Geometry check sheet. Reference: the model listing, model coordinates, mm. Face numbers are marked on the shaded views. Round coordinates to 2 decimals unless told otherwise and drop trailing zeros. Write each loop counter-clockwise with the first axis right and the second up, starting at its lowest first coordinate (ties: lowest second). Pieces come first, ordered by that corner, then holes.
Item 1: Cross-section at A-A (y = 3.5). Enter the section's corners in (x, z).
Item 2: Scan lines: probe 1 along X at (y, z) = (4.5, 6.75); probe 2 along Y at (x, z) = (25, 2.75); probe 3 along Y at (x, z) = (36.5, 2.5). Record each from-to range of solid material in increasing order.
Item 3: Depth check by flat-ended pin: P1, Ø1, axis at x = 8, y = 3, coming from the -Z side. Enter the tip coordinate at first touch or a pass-through.
Item 4: Draft check along Z on the marked faces 1, 2 and 3. Enter one of: pulls with the +Z half, pulls with the -Z half, needs draft (parallel to the pull), parting line crosses it, or undercut.
Item 5: Cross-section at C-C (x = 35). Enter the section's corners in (y, z).
Item 6: Cross-section at B-B (z = 3.5). Enter the section's corners in (x, y), then the cut area to 3 significant figures.
Item 7: Cross-section at D-D (z = 0.5). Enter the section's corners in (x, y), then the cut area to 3 significant figures.
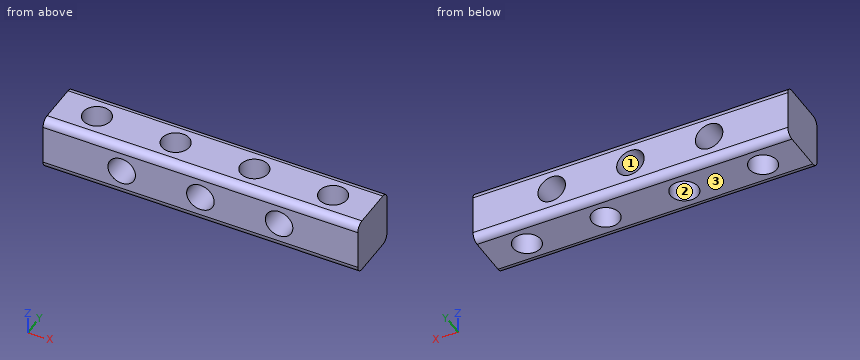
from build123d import *

# Parameters (mm, degrees)
SKETCH_1_W          = 40
SKETCH_1_H          = 7
SKETCH_1_R          = 1.75
EXTRUDE_1_DEPTH     = 7
SKETCH_2_R          = 1.75
CUT_EXTRUDE_1_DEPTH = 7
FILLET_1_R          = 1


with BuildPart() as part:
    # 草图1 → 凸台-拉伸1 (new body)
    with BuildSketch(Plane.XY):
        with Locations((20, 3.5)):
            Rectangle(SKETCH_1_W, SKETCH_1_H)
        with Locations((5, 3.5)):
            Circle(SKETCH_1_R, mode=Mode.SUBTRACT)
        with Locations((15, 3.5)):
            Circle(SKETCH_1_R, mode=Mode.SUBTRACT)
        with Locations((25, 3.5)):
            Circle(SKETCH_1_R, mode=Mode.SUBTRACT)
        with Locations((35, 3.5)):
            Circle(SKETCH_1_R, mode=Mode.SUBTRACT)
    extrude(amount=EXTRUDE_1_DEPTH)

    # 草图2 → 切除-拉伸1 (cut)
    with BuildSketch(Plane(origin=(0, 7, 0), x_dir=(1, 0, 0), z_dir=(0, 1, 0))):
        with Locations(Location((20, -3.5, 0), (0, 0, 270))):
            Circle(SKETCH_2_R)
        with Locations(Location((30, -3.5, 0), (0, 0, 270))):
            Circle(SKETCH_2_R)
        with Locations(Location((10, -3.5, 0), (0, 0, 270))):
            Circle(SKETCH_2_R)
    extrude(amount=-CUT_EXTRUDE_1_DEPTH, mode=Mode.SUBTRACT)

    # 圆角1
    fillet_1_edges = [part.edges().sort_by_distance(p)[0] for p in [
        (20, 7, 7),
        (20, 7, 0),
        (20, 0, 0),
        (20, 0, 7),
    ]]
    fillet(fillet_1_edges, radius=FILLET_1_R)


solid = part.part
Resolved:
1. outline: (0, 0) - (3.25, 0) - (3.25, 7) - (0, 7) - close; (6.75, 0) - (13.25, 0) - (13.25, 7) - (6.75, 7) - close; (16.75, 0) - (23.25, 0) - (23.25, 7) - (16.75, 7) - close; (26.75, 0) - (33.25, 0) - (33.25, 7) - (26.75, 7) - close; (36.75, 0) - (40, 0) - (40, 7) - (36.75, 7) - close; hole circle Ø3.5 at (10, 3.5); hole circle Ø3.5 at (20, 3.5); hole circle Ø3.5 at (30, 3.5)
2. probe 1: x = 0 to 3.56, 6.44 to 13.56, 16.44 to 23.56, 26.44 to 33.56, 36.44 to 40
2. probe 2: y = 0 to 1.75, 5.25 to 7
2. probe 3: y = 0 to 2.6, 4.4 to 7
3. P1: stops at z = 0
4. face 1: undercut
4. face 2: needs draft
4. face 3: pulls with the -Z half
5. outline: (0, 1) arc R1 ccw to (1, 0) - (1.75, 0) - (1.75, 7) - (1, 7) arc R1 ccw to (0, 6) - close; (5.25, 0) - (6, 0) arc R1 ccw to (7, 1) - (7, 6) arc R1 ccw to (6, 7) - (5.25, 7) - close
6. outline: (0, 0) - (8.25, 0) - (8.25, 7) - (0, 7) - close; (11.75, 0) - (18.25, 0) - (18.25, 7) - (11.75, 7) - close; (21.75, 0) - (28.25, 0) - (28.25, 7) - (21.75, 7) - close; (31.75, 0) - (40, 0) - (40, 7) - (31.75, 7) - close; hole circle Ø3.5 at (5, 3.5); hole circle Ø3.5 at (15, 3.5); hole circle Ø3.5 at (25, 3.5); hole circle Ø3.5 at (35, 3.5)
6. area: 168 mm2
7. outline: (0, 0.13) - (40, 0.13) - (40, 6.87) - (0, 6.87) - close; hole circle Ø3.5 at (5, 3.5); hole circle Ø3.5 at (15, 3.5); hole circle Ø3.5 at (25, 3.5); hole circle Ø3.5 at (35, 3.5)
7. area: 231 mm2
